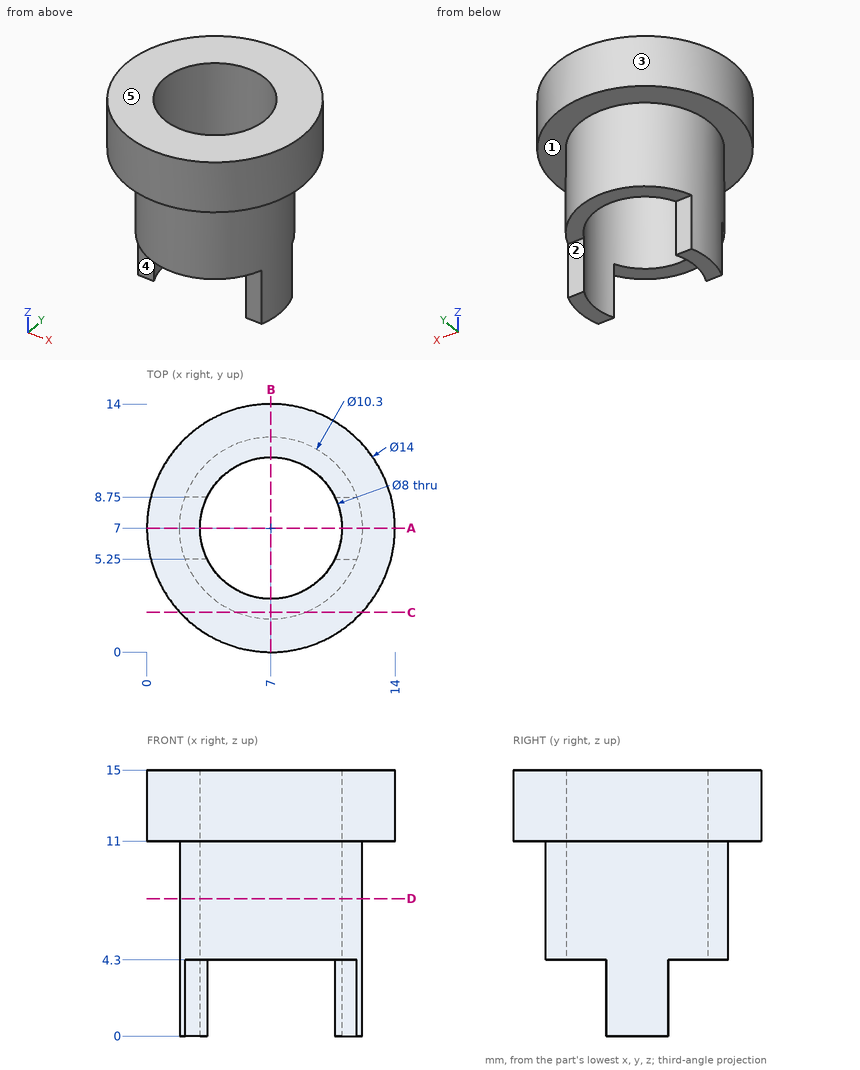
Design review of the part shown in the three views and the two pictorial views. Dimensions are in mm from the part's minimum x, y and z. A direction names the side the tool comes from. Coordinates: 2 decimals unless noted, no trailing zeros. Order: outer loops, then holes, each group sorted by start corner. A loop starts at its lowest first (then second) coordinate and runs counter-clockwise, first axis right, second up.
Item 1: For line 1 (Y direction, x = 7, z = 7); line 2 (Y direction, x = 8.75, z = 9.75), list the stretches that pass through material, from the lowest coordinate up.
Item 2: For pin 1 Ø1 at (x, z) = (2.5, 1.5) entering from -Y; pin 2 Ø0.6 at (x, z) = (11.5, 3) entering from -Y; pin 3 Ø1.5 at (x, z) = (12, 8.5) entering from +Y, all flat-tipped, find the tip position at first contact; note any pin that passes through.
Item 3: For the marked faces 1, 2, 3, 4 and 5, list the 3-axis set-ups (+Z, -Z, +X, -X, +Y, -Y) from which the entire face can be reached by the end or side of a thin tool; tool diameter is ignored.
Item 4: Take a section at D-D, the plane z = 7.75. Write out the cut boundary in (x, y).
Item 5: Take a section at A-A, the plane y = 7. Write out the cut boundary in (x, z), then the cut area to 3 significant figures.
Item 6: Take a section at B-B, the plane x = 7. Write out the cut boundary in (y, z), then the cut area to 3 significant figures.
Item 7: Take a section at C-C, the plane y = 2.25. Write out the cut boundary in (x, z).
The answers:
1. line 1: y = 1.85 to 3, 11 to 12.15
1. line 2: y = 2.16 to 3.4, 10.6 to 11.84
2. pin 1: stops at y = 5.25
2. pin 2: stops at y = 5.25
2. pin 3: stops at y = 9.91
3. face 1: -Z
3. face 2: -Z, +X, -X, +Y
3. face 3: +Z, -Z
3. face 4: -Z, +X, -X, -Y
3. face 5: +Z, +X, -X, +Y, -Y
4. outline: circle Ø10.3 at (7, 7); hole circle Ø8 at (7, 7)
5. outline: (0, 11) - (1.85, 11) - (1.85, 0) - (3, 0) - (3, 15) - (0, 15) - close; (11, 0) - (12.15, 0) - (12.15, 11) - (14, 11) - (14, 15) - (11, 15) - close
5. area: 49.3 mm2
6. outline: (0, 11) - (1.85, 11) - (1.85, 4.3) - (3, 4.3) - (3, 15) - (0, 15) - close; (11, 4.3) - (12.15, 4.3) - (12.15, 11) - (14, 11) - (14, 15) - (11, 15) - close
6. area: 39.4 mm2
7. outline: (1.86, 11) - (5.01, 11) - (5.01, 4.3) - (8.99, 4.3) - (8.99, 11) - (12.14, 11) - (12.14, 15) - (1.86, 15) - close
